The model under review builds one solid part; all positions refer to its coordinate system, in mm. Face numbers are marked on the shaded views. A direction names the side the tool comes from. Round coordinates to 2 decimals unless told otherwise and drop trailing zeros. Order: outer loops, then holes, each group sorted by start corner. A loop starts at its lowest first (then second) coordinate and runs counter-clockwise, first axis right, second up.
1) Consider section A-A (x = -15). Give the boundary of the cut face in (y, z), then the cut area to 3 significant figures.
2) Clearance check with flat-ended pins moving along their axes: P1, Ø4, axis at x = -17.96, y = 1.26, coming from the +Z side; P2, Ø2, axis at y = 0, z = -1, coming from the -X side; P3, Ø2, axis at x = -0.5, z = -2.5, coming from the +Y side. State where each tip first meets the part, or that it passes through.
3) To check wall thickness, follow L1, parallel to Y at x = 6.5, z = -3.45; L2, parallel to X at y = -12.5, z = -1.3; L3, parallel to Y at x = -6, z = -0.7. State the ranges of each line that lie inside material, in increasing order.
4) Mouldability with a two-part tool opening along Y and no side actions: class the marked faces 3, 4, 5 and 6 as pulls with the +Y half, pulls with the -Y half, needs draft (parallel to the pull), parting line crosses it, or undercut.
5) Machinability: for the marked faces 1 and 2, which of the approach directions +Z, -Z, +X, -X, +Y, -Y give a long, thin tool a straight path to every point of the face, cutting with its end or side? Answer none if there is none.
6) Consider section B-B (z = -1.4). Give the number of separate pieces and of enclosed holes in the cut face, then the cut area to 3 significant figures.
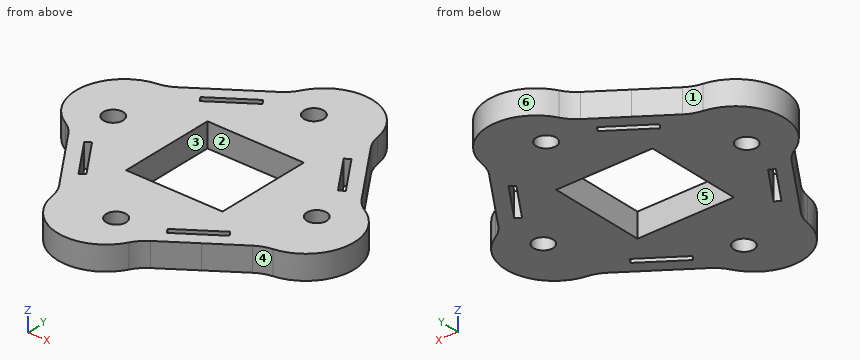
from build123d import *

# Parameters (mm, degrees)
PAD006_DEPTH          = 4
POLARPATTERN002_COUNT = 4
SKETCH012_W           = 16
SKETCH012_H           = 16
POCKET001_DEPTH       = 4.001
SKETCH018_R           = 1.65
HOLE_DEPTH            = 12.001
POCKET005_DEPTH       = 149.7520027338
POLARPATTERN_COUNT    = 4


with BuildPart() as part:
    # Sketch → Pad006 (new body)
    with BuildSketch(Plane.XY):
        with BuildLine():
            ThreePointArc((18.9209111487, -11.036007045), (25.6050015783, -4.5148526193), (21.5543772962, 3.8991216402))
            ThreePointArc((19.510343337, 5.7262546507), (20.4266011455, 4.694374188), (21.5543772962, 3.8991216402))
            Line((19.510343337, 5.7262546507), (15.7820965007, 11.0507429386))
            Line((0, 0), (15.7820965007, 11.0507429386))
            Line((0, 0), (11.0507429386, -15.7820965007))
            Line((11.0507429386, -15.7820965007), (16.3752312264, -12.0538496644))
            ThreePointArc((18.9209111487, -11.036007045), (17.5891558316, -11.3975778351), (16.3752312264, -12.0538496644))
        make_face()
    pad006 = extrude(amount=-PAD006_DEPTH)

    # PolarPattern002: Pad006 ×4 about axis
    polarpattern002_axis = Axis((0, 0, 0), (0, 0, 1))
    for i in range(1, POLARPATTERN002_COUNT):
        add(pad006.rotate(polarpattern002_axis, i * 360 / POLARPATTERN002_COUNT))

    # Sketch012 → Pocket001 (cut, through all)
    with BuildSketch(Plane.XY):
        Rectangle(SKETCH012_W, SKETCH012_H)
    extrude(amount=-POCKET001_DEPTH, mode=Mode.SUBTRACT)

    # Sketch018 → Hole (cut, through all)
    with BuildSketch(Plane.XY.offset(8)):
        with Locations((1.2556165274, 17.9561529047)):
            Circle(SKETCH018_R)
        with Locations((-1.2556165274, -17.9561529047)):
            Circle(SKETCH018_R)
        with Locations((-17.9561529047, 1.2556165274)):
            Circle(SKETCH018_R)
        with Locations((17.9561529047, -1.2556165274)):
            Circle(SKETCH018_R)
    extrude(amount=-HOLE_DEPTH, mode=Mode.SUBTRACT)

    # Sketch021 → Pocket005 (cut, through all)
    with BuildSketch(Plane.XY):
        Polygon((11.2159688683, 12.0143126733), (12.0351209126, 12.5878891096), (16.6237324034, 6.0346727553), (15.8045803591, 5.461096319), align=None)
    pocket005 = extrude(amount=-POCKET005_DEPTH, mode=Mode.SUBTRACT)

    # PolarPattern: Pocket005 ×4 about axis
    polarpattern_axis = Axis((0, 0, 0), (0, 0, 1))
    for i in range(1, POLARPATTERN_COUNT):
        add(pocket005.rotate(polarpattern_axis, i * 360 / POLARPATTERN_COUNT), mode=Mode.SUBTRACT)


solid = part.part
Answer below:
1. outline: (-12.17, -4) - (-8.35, -4) - (-8.35, 0) - (-12.17, 0) - close; (-6.61, -4) - (13.02, -4) - (13.02, 0) - (-6.61, 0) - close
1. area: 93.8 mm2
2. P1: stops at z = 0
2. P2: stops at x = -25.44
2. P3: stops at y = 25.28
3. L1: y = -18.97 to -16.3, -15.08 to -8, 8 to 24.98
3. L2: x = -14.77 to -12.1, -11.91 to 10.18, 11.92 to 15.74
3. L3: y = -25.19 to -8, 8 to 15.43, 16.57 to 19.32
4. face 3: undercut
4. face 4: pulls with the -Y half
4. face 5: undercut
4. face 6: pulls with the +Y half
5. face 1: +Z, -Z, -X, +Y
5. face 2: +Z, -Z
6. separate pieces: 1
6. enclosed holes: 9
6. area: 1,230 mm2
